Design review of the part built by this model. Coordinates are the model's own, in mm. A direction names the side the tool comes from. Coordinates: 2 decimals unless noted, no trailing zeros. Write each loop counter-clockwise with the first axis right and the second up, starting at its lowest first coordinate (ties: lowest second). Pieces come first, ordered by that corner, then holes.
Q1. Take a section at A-A (y = 12.5). Give the boundary of the cut face in (x, z) (3 decimals), and give its area (3 significant figures).
Q2. Take a section at B-B (z = 15.5). Give the boundary of the cut face in (x, y).
Q3. For probe 1 along X at (y, z) = (3, 4); probe 2 along Y at (x, z) = (11.5, 5); probe 3 along X at (y, z) = (6, 4.25), list the stretches that pass through material, from the lowest coordinate up.
Q4. Take a section at C-C (x = 4.75). Give the boundary of the cut face in (y, z) (3 decimals).
Q5. Machinability: for faces 4 (the flat face through (0, 0.6, 16)), 5 (the flat face through (-5, 11, 6.65)), 6 (the flat face through (0, 1.3, 16)), 7 (the flat face through (-5, 11, 0.3)), 8 (the cylindrical face through (10.953, 1.001, 2.17)), which of the approach directions +Z, -Z, +X, -X, +Y, -Y give a long, thin tool a straight path to every point of the face, cutting with its end or side? Answer none if there is none.
Q6. Insertion check: pin 1 (5 mm diameter, centred on x = 5, y = 9, fed in from +Z); pin 2 (1.5 mm diameter, centred on x = -7.5, y = 3.5, fed in from -Z); pin 3 (7 mm diameter, centred on y = 11, z = 4.5, fed in from -X); pin 4 (3 mm diameter, centred on y = 10.5, z = 4, fed in from +X). Each pin has a flat end and moves straight along its axis. Give the tip position at first contact, or say it passes through.
Q7. Take a section at D-D (y = 10). Give the boundary of the cut face in (x, z), and give its area (3 significant figures).
Q8. Mouldability with a two-part tool opening along Z and no side actions: class faces 1 (the flat face through (-2.5, 11, 3)), 2 (the flat face through (5, 11, 0.3)), 3 (the flat face through (5, 13, 3.075)) as pulls with the +Z half, pulls with the -Z half, needs draft (parallel to the pull), parting line crosses it, or undercut.
```python
from build123d import *

# Parameters (mm, degrees)
SKETCH1_W                = 26.2
SKETCH1_H                = 7.2
SKETCH1_R                = 1.6
BOSS_EXTRUDE1_DEPTH      = 6.95
BOSS_EXTRUDE2_DEPTH      = 3.175
BOSS_EXTRUDE2_DEPTH_BACK = 3.175
SKETCH2_W                = 4.2
SKETCH2_H                = 8.3
SKETCH3_W                = 0.8
SKETCH3_H                = 2
CUT_EXTRUDE1_DEPTH       = 27.088167816
SKETCH4_W                = 13.4
SKETCH4_H                = 6.2
BOSS_EXTRUDE3_DEPTH      = 7.55
SKETCH5_W                = 13
SKETCH5_H                = 0.7
BOSS_EXTRUDE4_DEPTH      = 3.8
SKETCH6_W                = 11.057539052
SKETCH6_H                = 0.3
BOSS_EXTRUDE5_DEPTH      = 6.2
SKETCH7_R                = 0.35
SKETCH7_W                = 0.673728729
SKETCH7_H                = 6.2
SKETCH7_W_2              = 0.592367936
SKETCH7_W_3              = 0.568302757
SKETCH7_W_4              = 0.558499764
SKETCH7_W_5              = 0.793155974
CUT_EXTRUDE3_DEPTH       = 2
CUT_EXTRUDE4_DEPTH       = 26.864841001
SKETCH10_W               = 3
SKETCH10_H               = 3
BOSS_EXTRUDE6_DEPTH      = 0.2


with BuildPart() as part:
    # Sketch1 → Boss-Extrude1 (new body)
    with BuildSketch(Plane.XY):
        with Locations((0, 3.6)):
            Rectangle(SKETCH1_W, SKETCH1_H)
        with Locations((-10.311776953, 3.6)):
            Circle(SKETCH1_R, mode=Mode.SUBTRACT)
        with Locations(Location((10.311776953, 3.6, 0), (0, 0, 180))):
            Circle(SKETCH1_R, mode=Mode.SUBTRACT)
    extrude(amount=BOSS_EXTRUDE1_DEPTH)

    # Sketch2 → Boss-Extrude2 (add, two sides: drawn at the far end of the back side and taken through both)
    with BuildSketch(Plane.XY.offset(3.475).offset(-BOSS_EXTRUDE2_DEPTH_BACK)):
        with Locations((-4.6, 11.35)):
            Rectangle(SKETCH2_W, SKETCH2_H)
        with Locations((4.6, 11.35)):
            Rectangle(SKETCH2_W, SKETCH2_H)
    extrude(amount=BOSS_EXTRUDE2_DEPTH + BOSS_EXTRUDE2_DEPTH_BACK)

    # Sketch3 → Cut-Extrude1 (cut, through all)
    with BuildSketch(Plane.ZY.offset(6.7)):
        with Locations((3.475, 12.64)):
            Rectangle(SKETCH3_W, SKETCH3_H)
    extrude(amount=-CUT_EXTRUDE1_DEPTH, mode=Mode.SUBTRACT)

    # Sketch4 → Boss-Extrude3 (add)
    with BuildSketch(Plane.XY.offset(6.95)):
        with Locations((0, 3.1)):
            Rectangle(SKETCH4_W, SKETCH4_H)
    extrude(amount=BOSS_EXTRUDE3_DEPTH)

    # Sketch5 → Boss-Extrude4 (add)
    with BuildSketch(Plane.XY.offset(14.5)):
        with Locations((0, 0.95)):
            Rectangle(SKETCH5_W, SKETCH5_H)
    extrude(amount=BOSS_EXTRUDE4_DEPTH)

    # Sketch6 → Boss-Extrude5 (add)
    with BuildSketch(Plane.XY.offset(14.5)):
        with Locations((0, 3.95)):
            Rectangle(SKETCH6_W, SKETCH6_H)
    extrude(amount=BOSS_EXTRUDE5_DEPTH)

    # Sketch7 → Cut-Extrude3 (cut)
    with BuildSketch(Plane(origin=(0, 4.1, 0), x_dir=(1, 0, 0), z_dir=(0, 1, 0))):
        Polygon((-5.219979377, -20.517795083), (-5.219979377, -14.5), (-5.528769526, -14.5), (-5.528769526, -20.7), (-5.219979377, -20.7), align=None)
        with Locations(Location((-4.273866855, -19.926328783, 0), (0, 0, 180))):
            Circle(SKETCH7_R)
        with Locations((-3.221250813, -17.6)):
            Rectangle(SKETCH7_W, SKETCH7_H)
        with Locations((-2.58820248, -17.6)):
            Rectangle(SKETCH7_W_2, SKETCH7_H)
        with Locations(Location((-1.733866855, -19.926328783, 0), (0, 0, 180))):
            Circle(SKETCH7_R)
        with Locations((-0.681250813, -17.6)):
            Rectangle(SKETCH7_W, SKETCH7_H)
        with Locations((-0.06023507, -17.6)):
            Rectangle(SKETCH7_W_3, SKETCH7_H)
        with Locations((1.858749188, -17.6)):
            Rectangle(SKETCH7_W, SKETCH7_H)
        with Locations((2.474863434, -17.6)):
            Rectangle(SKETCH7_W_4, SKETCH7_H)
        with Locations((4.398749187, -17.6)):
            Rectangle(SKETCH7_W, SKETCH7_H)
        with Locations((5.132191539, -17.6)):
            Rectangle(SKETCH7_W_5, SKETCH7_H)
        with BuildLine():
            Line((-5.219979377, -20.7), (-5.03777446, -20.7))
            ThreePointArc((-5.03777446, -20.7), (-5.166612793, -20.646633415), (-5.219979377, -20.517795083))
            Line((-5.219979377, -20.517795083), (-5.219979377, -20.7))
        make_face()
        with Locations(Location((0.806133145, -19.926328783, 0), (0, 0, 180))):
            Circle(SKETCH7_R)
        with Locations(Location((3.346133145, -19.926328783, 0), (0, 0, 180))):
            Circle(SKETCH7_R)
    extrude(amount=-CUT_EXTRUDE3_DEPTH, mode=Mode.SUBTRACT)

    # Sketch9 → Cut-Extrude4 (cut, through all)
    with BuildSketch(Plane(origin=(0, 7.2, 0), x_dir=(1, 0, 0), z_dir=(0, 1, 0))):
        with BuildLine():
            Line((9.243559577, -4.896961438), (9.756440423, -4.896961438))
            ThreePointArc((9.756440423, -4.896961438), (10.939656379, -4.436341133), (11.5, -3.296961438))
            ThreePointArc((11.5, -3.296961438), (10.939656379, -2.157581742), (9.756440423, -1.696961438))
            Line((9.756440423, -1.696961438), (9.243559577, -1.696961438))
            ThreePointArc((9.243559577, -1.696961438), (8.060343621, -2.157581742), (7.5, -3.296961438))
            ThreePointArc((7.5, -3.296961438), (8.060343621, -4.436341133), (9.243559577, -4.896961438))
        make_face()
        with BuildLine():
            Line((-9.243559577, -4.896961438), (-9.756440423, -4.896961438))
            ThreePointArc((-9.756440423, -4.896961438), (-10.939656379, -4.436341133), (-11.5, -3.296961438))
            ThreePointArc((-11.5, -3.296961438), (-10.939656379, -2.157581742), (-9.756440423, -1.696961438))
            Line((-9.756440423, -1.696961438), (-9.243559577, -1.696961438))
            ThreePointArc((-9.243559577, -1.696961438), (-8.060343621, -2.157581742), (-7.5, -3.296961438))
            ThreePointArc((-7.5, -3.296961438), (-8.060343621, -4.436341133), (-9.243559577, -4.896961438))
        make_face()
    extrude(amount=-CUT_EXTRUDE4_DEPTH, mode=Mode.SUBTRACT)

    # Sketch10 → Boss-Extrude6 (add)
    with BuildSketch(Plane(origin=(0, 6.2, 0), x_dir=(1, 0, 0), z_dir=(0, 1, 0))):
        with Locations((-2.650474803, -8.66301906)):
            Rectangle(SKETCH10_W, SKETCH10_H)
    extrude(amount=BOSS_EXTRUDE6_DEPTH)


solid = part.part
```
Response:
1. outline: (-6.7, 0.3) - (-2.5, 0.3) - (-2.5, 3.075) - (-6.7, 3.075) - close; (-6.7, 3.875) - (-2.5, 3.875) - (-2.5, 6.65) - (-6.7, 6.65) - close; (2.5, 0.3) - (6.7, 0.3) - (6.7, 3.075) - (2.5, 3.075) - close; (2.5, 3.875) - (6.7, 3.875) - (6.7, 6.65) - (2.5, 6.65) - close
1. area: 46.6 mm2
2. outline: (-6.5, 0.6) - (6.5, 0.6) - (6.5, 1.3) - (-6.5, 1.3) - close; (-5.22, 3.8) - (-3.56, 3.8) - (-3.56, 4.1) - (-5.22, 4.1) - close; (-2.29, 3.8) - (-1.02, 3.8) - (-1.02, 4.1) - (-2.29, 4.1) - close; (0.22, 3.8) - (1.52, 3.8) - (1.52, 4.1) - (0.22, 4.1) - close; (2.75, 3.8) - (4.06, 3.8) - (4.06, 4.1) - (2.75, 4.1) - close
3. probe 1: x = -13.1 to -11.8, -7.72 to 7.72, 11.8 to 13.1
3. probe 2: y = 0 to 2.53, 4.67 to 7.2
3. probe 3: x = -13.1 to -11.12, -7.88 to 7.88, 11.12 to 13.1
4. outline: (0, 0) - (7.2, 0) - (7.2, 0.3) - (15.5, 0.3) - (15.5, 6.65) - (7.2, 6.65) - (7.2, 6.95) - (6.2, 6.95) - (6.2, 14.5) - (1.3, 14.5) - (1.3, 18.3) - (0.6, 18.3) - (0.6, 14.5) - (0, 14.5) - close; hole (11.64, 3.075) - (13.64, 3.075) - (13.64, 3.875) - (11.64, 3.875) - close
5. face 4: +Z, +X, -X, -Y
5. face 5: +Z, +X, -X, +Y
5. face 6: +Z, +X, -X
5. face 7: -Z, +X, -X, +Y
5. face 8: +Y, -Y
6. pin 1: stops at z = 6.95
6. pin 2: stops at z = 0
6. pin 3: stops at x = -6.7
6. pin 4: stops at x = 6.7
7. outline: (-6.7, 0.3) - (-2.5, 0.3) - (-2.5, 6.65) - (-6.7, 6.65) - close; (2.5, 0.3) - (6.7, 0.3) - (6.7, 6.65) - (2.5, 6.65) - close
7. area: 53.3 mm2
8. face 1: needs draft
8. face 2: pulls with the -Z half
8. face 3: undercut
